Here's how the part is built. I have some questions about the finished solid (model axes, mm). A direction names the side the tool comes from. Give positions to 0.01 mm unless a question says otherwise; leave off trailing zeros. Write each loop counter-clockwise with the first axis right and the second up, starting at its lowest first coordinate (ties: lowest second). Pieces come first, ordered by that corner, then holes. Notation, with made-up numbers: (72, 2) - (78, 2) arc R9 cw to (78, 17) - close; hole circle Ø2 at (-21.75, -24.75). An arc over 180 degrees is marked (long way). Use a Markdown table: item, result.
```python
from build123d import *

# Parameters (mm, degrees)
SKETCH1_W           = 130
SKETCH1_H           = 90
BOSS_EXTRUDE1_DEPTH = 5
FILLET1_R           = 20
SKETCH2_R           = 4
CUT_EXTRUDE1_DEPTH  = 3
SKETCH3_R           = 2
CUT_EXTRUDE2_DEPTH  = 6
SKETCH4_W           = 25
SKETCH4_H           = 35
BOSS_EXTRUDE2_DEPTH = 30


with BuildPart() as part:
    # Sketch1 → Boss-Extrude1 (new body)
    with BuildSketch(Plane.XY):
        Rectangle(SKETCH1_W, SKETCH1_H)
    extrude(amount=BOSS_EXTRUDE1_DEPTH)

    # Fillet1
    fillet1_edges = [part.edges().sort_by_distance(p)[0] for p in [
        (65, -45, 2.5),
        (-65, -45, 2.5),
        (-65, 45, 2.5),
        (65, 45, 2.5),
    ]]
    fillet(fillet1_edges, radius=FILLET1_R)

    # Sketch2 → Cut-Extrude1 (cut)
    with BuildSketch(Plane(origin=(0, 0, 0), x_dir=(-1, 0, 0), z_dir=(0, 0, -1))):
        with Locations((-39.142135624, 39.142135624)):
            Circle(SKETCH2_R)
        with Locations((39.142135624, 39.142135624)):
            Circle(SKETCH2_R)
        with Locations((-39.142135624, -39.142135624)):
            Circle(SKETCH2_R)
        with Locations((39.142135624, -39.142135624)):
            Circle(SKETCH2_R)
    extrude(amount=-CUT_EXTRUDE1_DEPTH, mode=Mode.SUBTRACT)

    # Sketch3 → Cut-Extrude2 (cut, through all)
    with BuildSketch(Plane(origin=(0, 0, 0), x_dir=(-1, 0, 0), z_dir=(0, 0, -1))):
        with Locations((-39.142135624, 39.142135624)):
            Circle(SKETCH3_R)
        with Locations((39.142135624, 39.142135624)):
            Circle(SKETCH3_R)
        with Locations((39.142135624, -39.142135624)):
            Circle(SKETCH3_R)
        with Locations((-39.142135624, -39.142135624)):
            Circle(SKETCH3_R)
    extrude(amount=-CUT_EXTRUDE2_DEPTH, mode=Mode.SUBTRACT)

    # Sketch4 → Boss-Extrude2 (add)
    with BuildSketch(Plane.XY.offset(5)):
        with Locations((-39.142135624, 0)):
            Rectangle(SKETCH4_W, SKETCH4_H)
    extrude(amount=BOSS_EXTRUDE2_DEPTH)


solid = part.part
```
Item 1: I need wall thicknesses on line 1 along X through (y, z) = (9.5, 32); line 2 along Z through (x, y) = (17.5, 34); line 3 along Y through (x, z) = (-32, 25.5). Which ranges of each line are inside material? Lowest first, please. Write a range as [from, to].
Values:
| item | result |
|---|---|
| line 1 | x = [-51.64, -26.64] |
| line 2 | z = [0, 5] |
| line 3 | y = [-17.5, 17.5] |
Item 2: For faces 4 (the flat face through (-51.642, 0, 20)), 5 (the flat face through (-26.642, 0, 20)), 6 (the flat face through (-39, 17.5, 20)), 7 (the flat face through (-39, -17.5, 20)), 8 (the flat face through (-40, -37, 3)), which set-ups out of +Z, -Z, +X, -X, +Y, -Y let a thin tool reach every point of the face, with its end or its side?
Values:
| item | result |
|---|---|
| face 4 | +Z, -X, +Y, -Y |
| face 5 | +Z, +X, +Y, -Y |
| face 6 | +Z, +X, -X, +Y |
| face 7 | +Z, +X, -X, -Y |
| face 8 | -Z |
Item 3: If we section it at B-B, the plane z = 15.5: Write out the boundary of the cut face in (x, y).
Values:
| item | result |
|---|---|
| outline | (-51.64, -17.5) - (-26.64, -17.5) - (-26.64, 17.5) - (-51.64, 17.5) - close |
Item 4: If we section it at C-C, the plane x = 7: Write out the boundary of the cut face in (y, z), plus the area to 3 significant figures.
Values:
| item | result |
|---|---|
| outline | (-45, 0) - (45, 0) - (45, 5) - (-45, 5) - close |
| area | 450 mm2 |
Item 5: Thinking about a two-plate mould opening in X: for faces 1 (the cylindrical face through (59.297, 38.986, 2.535)), 2 (the cylindrical face through (-42.837, 37.61, 1.479)), 3 (the flat face through (-1, 45, 2)), which applies, +X half, -X half, draft (parallel to the pull), parting line (faces both ways), or undercut?
Values:
| item | result |
|---|---|
| face 1 | +X half |
| face 2 | undercut |
| face 3 | draft |
Item 6: If we section it at A-A, the plane y = 13: Write out the boundary of the cut face in (x, z), plus the area to 3 significant figures.
Values:
| item | result |
|---|---|
| outline | (-65, 0) - (65, 0) - (65, 5) - (-26.64, 5) - (-26.64, 35) - (-51.64, 35) - (-51.64, 5) - (-65, 5) - close |
| area | 1,400 mm2 |
Item 7: Will these pins go through, and if not, where does the flat tip stop? pin 1 Ø5 at (x, z) = (51, 6) entering from +Y; pin 2 Ø10 at (x, y) = (35.5, 10) entering from +Z; pin 3 Ø12 at (x, y) = (25, 32.5) entering from -Z; pin 4 Ø5 at (x, y) = (39.14, -39.14) entering from -Z.
Values:
| item | result |
|---|---|
| pin 1 | stops at y = 44.65 |
| pin 2 | stops at z = 5 |
| pin 3 | stops at z = 0 |
| pin 4 | stops at z = 3 |
